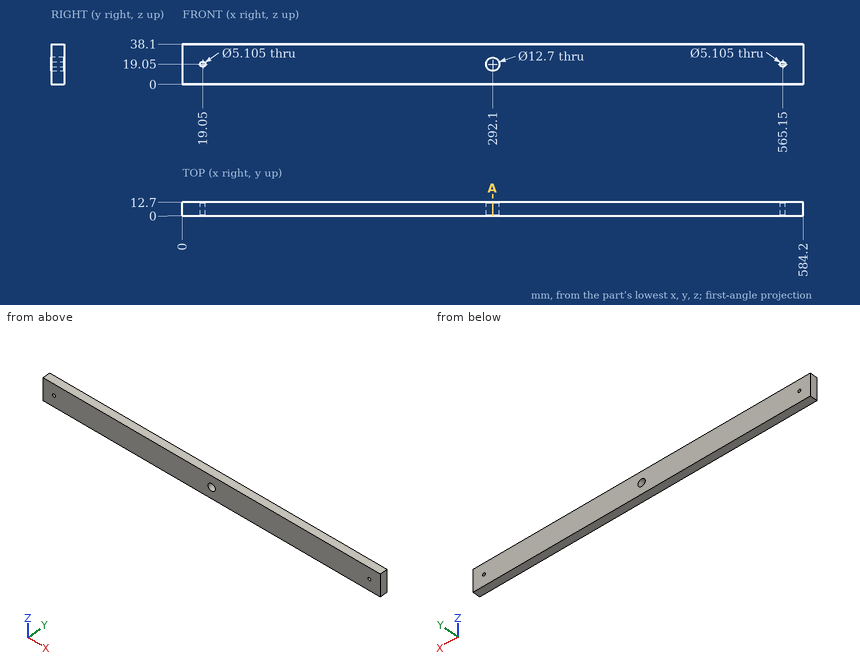
The figure shows three views and two pictorial views of one solid part (mm, origin at its lowest corner). Answer the questions. Give positions to 0.01 mm unless a question says otherwise; leave off trailing zeros. Order: outer loops, then holes, each group sorted by start corner. A loop starts at its lowest first (then second) coordinate and runs counter-clockwise, first axis right, second up. Notation, with made-up numbers: (88.25, 73) - (137.25, 73) arc R20 ccw to (137.25, 98) - close; hole circle Ø7 at (-31.5, 71.5). An arc over 180 degrees is marked (long way). Answer as CSV lines item,"result".
Q1. Straight lines are drawn through the part: L1, parallel to X at y = 7.25, z = 19.05; L2, parallel to Z at x = 292.1, y = 4; L3, parallel to Z at x = 565.15, y = 9.75. For each, find the intervals that lie inside material, in ascending order.
Answer key:
L1,"x = 0 to 16.5, 21.6 to 285.75, 298.45 to 562.6, 567.7 to 584.2"
L2,"z = 0 to 12.7, 25.4 to 38.1"
L3,"z = 0 to 16.5, 21.6 to 38.1"
Q2. This flat-tipped pin is pushed along its axis until it touches: pin 1 Ø3 at (x, z) = (565.15, 19.05) entering from +Y. Where does it stop, or does it pass through?
Answer key:
pin 1,"passes through"
Q3. A cutting plane is placed at A-A, the plane x = 292.1. Determine the outline of the cut face in (y, z).
Answer key:
outline,"(0, 0) - (12.7, 0) - (12.7, 12.7) - (0, 12.7) - close; (0, 25.4) - (12.7, 25.4) - (12.7, 38.1) - (0, 38.1) - close"
